CAD build for the part. Positions are in the model's coordinates, mm. Face numbers are marked on the shaded views. A direction names the side the tool comes from. Give positions to 0.01 mm unless a question says otherwise; leave off trailing zeros. Loops run counter-clockwise (first coordinate to the right, second up) from the corner with the lowest first, then second, coordinate; pieces in that order, holes last. Notation, with made-up numbers: (-5.5, 38) - (34.5, 38) arc R14 cw to (34.5, 54) - close; hole circle Ø2 at (-17.75, 71.5). An arc over 180 degrees is marked (long way). Return JSON: item names as keys, results as strings.
from build123d import *

# Parameters (mm, degrees)
SKETCH1_W            = 36.3
SKETCH1_H            = 17
SKETCH1_W_2          = 22.3
SKETCH1_H_2          = 9
BOSS_EXTRUDE1_DEPTH  = 8.75
M3_CLEARANCE_HOLE1_D = 3.6
FILLET1_R            = 2


with BuildPart() as part:
    # Sketch1 → Boss-Extrude1 (new body)
    with BuildSketch(Plane(origin=(0, 0, 0), x_dir=(1, 0, 0), z_dir=(0, 1, 0))):
        with Locations((18.15, 8.5)):
            Rectangle(SKETCH1_W, SKETCH1_H)
        with Locations((18.15, 8.5)):
            Rectangle(SKETCH1_W_2, SKETCH1_H_2, mode=Mode.SUBTRACT)
    extrude(amount=BOSS_EXTRUDE1_DEPTH)

    # M3 Clearance Hole1 (through all)
    with Locations(Plane(origin=(0, 8.75, 0), x_dir=(1, 0, 0), z_dir=(0, 1, 0))):
        with Locations((3.050005, 3.4), (33.050005, -1.6), (33.050005, 13.4), (3.050005, 13.4)):
            Hole(M3_CLEARANCE_HOLE1_D / 2)

    # Fillet1
    fillet1_edges = [part.edges().sort_by_distance(p)[0] for p in [
        (0, 4.375, -17),
        (36.3, 4.375, -17),
        (36.3, 4.375, 0),
        (0, 4.375, 0),
    ]]
    fillet(fillet1_edges, radius=FILLET1_R)


solid = part.part
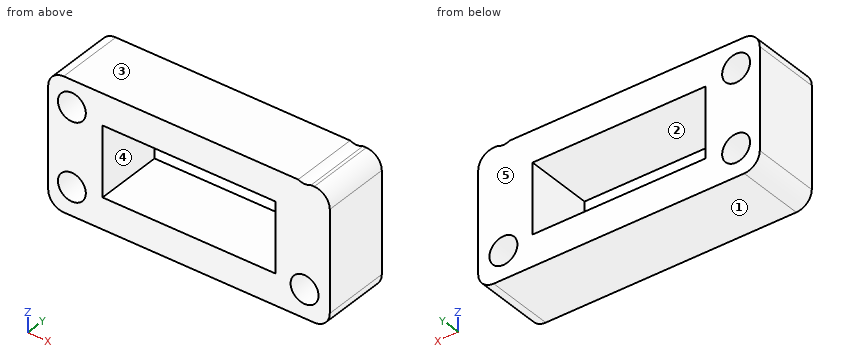
1. Pull direction Z, two halves, no side cores. Call the marked faces 1, 2 and 3: +Z half, -Z half, draft (parallel to the pull), parting line (faces both ways), or undercut.
Values follow:
{"face 1": "-Z half", "face 2": "undercut", "face 3": "+Z half"}
2. Cut at D-D, the plane z = -13.4. Write the cut outline in (x, y), plus the area to 3 significant figures.
Values follow:
{"outline": "(0, 0) - (1.25, 0) - (1.25, 8.75) - (0, 8.75) - close; (4.85, 0) - (31.25, 0) - (31.25, 8.75) - (4.85, 8.75) - close; (34.85, 0) - (36.3, 0) - (36.3, 8.75) - (34.85, 8.75) - close", "area": "255 mm²"}
3. Cut at C-C, the plane y = 4.5. Write the cut outline in (x, z).
Values follow:
{"outline": "(0, -15) arc R2 ccw to (2, -17) - (34.3, -17) arc R2 ccw to (36.3, -15) - (36.3, -2) arc R2 ccw to (34.3, 0) - (33.87, 0) arc R1.8 cw to (32.23, 0) - (2, 0) arc R2 ccw to (0, -2) - close; hole circle Ø3.6 at (3.05, -13.4); hole circle Ø3.6 at (3.05, -3.4); hole (7, -13) - (29.3, -13) - (29.3, -4) - (7, -4) - close; hole circle Ø3.6 at (33.05, -13.4)"}
4. Drop flat-ended pins along their axis: P1, Ø5, axis at x = 15.5, z = -7, coming from the -Y side; P2, Ø4.5, axis at x = 3.05, z = -3.4, coming from the +Y side. Give the stop position or say it passes through.
Values follow:
{"P1": "passes through", "P2": "stops at y = 8.75"}
5. Which spindle directions (+Z, -Z, +X, -X, +Y, -Y) get a long thin tool onto all of the face, cutting with end or side? Do the marked faces 4 and 5. Say none if no direction does.
Values follow:
{"face 4": "+Y, -Y", "face 5": "+Z, -Z, +X, -X, +Y"}
6. Cut at B-B, the plane z = -9. Write the cut outline in (x, y).
Values follow:
{"outline": "(0, 0) - (7, 0) - (7, 8.75) - (0, 8.75) - close; (29.3, 0) - (36.3, 0) - (36.3, 8.75) - (29.3, 8.75) - close"}
7. Cut at A-A, the plane x = 13. Write the cut outline in (y, z), plus the area to 3 significant figures.
Values follow:
{"outline": "(0, -17) - (8.75, -17) - (8.75, -13) - (0, -13) - close; (0, -4) - (8.75, -4) - (8.75, 0) - (0, 0) - close", "area": "70.0 mm²"}
8. Drill centre lines: probe 1 along X at (y, z) = (7.25, -13.4); probe 2 along Z at (x, y) = (24.5, 4.5); probe 3 along X at (y, z) = (1, -11.5). Where is each one in solid material? Low to high.
Values follow:
{"probe 1": "x = 0 to 1.25, 4.85 to 31.25, 34.85 to 36.3", "probe 2": "z = -17 to -13, -4 to 0", "probe 3": "x = 0 to 7, 29.3 to 36.3"}
